from build123d import *

# Parameters (mm, degrees)
F0_W        = 86.36
F0_H        = 24.892
F0_W_2      = 73.66
F0_H_2      = 12.192
F1_DEPTH    = 19.05
F1_FACE_W   = 86.36
F1_FACE_H   = 24.892
F1_FACE_W_2 = 73.66
F1_FACE_H_2 = 12.192
F2_DEPTH    = 12.7
F3_W        = 2.54
F3_H        = 12.192
F3_W_2      = 5.08
F4_DEPTH    = 6.35
F3_W_3      = 86.36
F3_H_2      = 24.892
F5_DEPTH    = 12.7
F7_W        = 73.66
F7_H        = 12.192
F8_DEPTH    = 2.54
F6_W        = 73.66
F6_H        = 3.81
F9_DEPTH    = 18.542


with BuildPart() as f1:
    # F0 (on Top) → F1 (new body)
    with BuildSketch(Plane.XY):
        Rectangle(F0_W, F0_H)
        Rectangle(F0_W_2, F0_H_2, mode=Mode.SUBTRACT)
    extrude(amount=F1_DEPTH)

    # F1_face (on face) → F2 (join)
    with BuildSketch(Plane(origin=(0, 0, 0), x_dir=(1, 0, 0), z_dir=(0, 0, -1))):
        Rectangle(F1_FACE_W, F1_FACE_H)
        Rectangle(F1_FACE_W_2, F1_FACE_H_2, mode=Mode.SUBTRACT)
    extrude(amount=F2_DEPTH)

    # F3 (on face) → F4 (join)
    with BuildSketch(Plane(origin=(0, 0, -12.7), x_dir=(1, 0, 0), z_dir=(0, 0, -1))):
        with Locations((-31.75, 0)):
            Rectangle(F3_W, F3_H)
        Rectangle(F3_W_2, F3_H)
        with Locations((31.75, 0)):
            Rectangle(F3_W, F3_H)
    extrude(amount=-F4_DEPTH)

    # F3 (on face) → F5 (join)
    with BuildSketch(Plane(origin=(0, 0, -12.7), x_dir=(1, 0, 0), z_dir=(0, 0, -1))):
        Rectangle(F3_W_3, F3_H_2)
        Polygon((-2.54, 6.096), (2.54, 6.096), (30.48, 6.096), (33.02, 6.096), (36.83, 6.096), (36.83, -6.096), (33.02, -6.096), (30.48, -6.096), (2.54, -6.096), (-2.54, -6.096), (-30.48, -6.096), (-33.02, -6.096), (-36.83, -6.096), (-36.83, 6.096), (-33.02, 6.096), (-30.48, 6.096), align=None, mode=Mode.SUBTRACT)
    extrude(amount=F5_DEPTH)

    # F7 (on face) → F8 (join)
    with BuildSketch(Plane(origin=(0, 0, -25.4), x_dir=(1, 0, 0), z_dir=(0, 0, -1))):
        Rectangle(F7_W, F7_H)
    extrude(amount=-F8_DEPTH)

    # F6 (on face) → F9 (cut)
    with BuildSketch(Plane.XZ.offset(12.446)):
        with Locations((0, -22.225)):
            Rectangle(F6_W, F6_H)
    extrude(amount=-F9_DEPTH, mode=Mode.SUBTRACT)


solid = f1.part
Here's how the part is built. I have some questions about the finished solid (model axes, mm). A direction names the side the tool comes from. Coordinates: 2 decimals unless noted, no trailing zeros. Order: outer loops, then holes, each group sorted by start corner. A loop starts at its lowest first (then second) coordinate and runs counter-clockwise, first axis right, second up. Notation, with made-up numbers: M 30,-25 L 67,-25 A15 cw 67,-8 Z; hole C 1,87 d1. An arc over 180 degrees is marked long. Answer as CSV lines item,"result".
Item 1: For pin 1 (1 mm diameter, centred on x = -29.5, y = -1, fed in from +Z); pin 2 (1.3 mm diameter, centred on x = -31.5, y = -2.5, fed in from +Z), each with a flat end and sliding along its axis, tell me the tip position at first contact or that it passes through.
Results found:
pin 1,"z = -24.13"
pin 2,"z = -6.35"
Item 2: Imagine slicing it at D-D on x = 0.5. Write out the boundary of the cut face in (y, z), plus the area to 3 significant figures.
Results found:
outline,"M -12.45,-25.4 L 12.45,-25.4 L 12.45,19.05 L 6.1,19.05 L 6.1,-6.35 L -6.1,-6.35 L -6.1,19.05 L -12.45,19.05 L -12.45,-20.32 L -6.1,-20.32 L -6.1,-12.7 L 6.1,-12.7 L 6.1,-24.13 L -12.45,-24.13 Z"
area,"633 mm2"
Item 3: Imagine slicing it at B-B on x = 12. Write out the boundary of the cut face in (y, z), plus the area to 3 significant figures.
Results found:
outline,"M -12.45,-25.4 L 12.45,-25.4 L 12.45,19.05 L 6.1,19.05 L 6.1,-24.13 L -12.45,-24.13 Z; M -12.45,-20.32 L -6.1,-20.32 L -6.1,19.05 L -12.45,19.05 Z"
area,"556 mm2"
Item 4: On a 3-axis mill with a long thin cutter (end or side, diameter ignored), from which of +Z, -Z, +X, -X, +Y, -Y can I reach the whole of each face in a straight line? I mean faces 1 (the face through (33.02, 0, -10)), 2 (the face through (-32, 0, -12.7)), 3 (the face through (-1, 8, 19.05)). Say none if no direction works.
Results found:
face 1,"+Z"
face 2,"none"
face 3,"+Z, +X, -X, +Y, -Y"
Item 5: If I drill on line 1 (X direction, y = -3, z = -11); line 2 (Z direction, x = 1.5, y = -5); line 3 (Y direction, x = -4, z = -5.5), over which ranges is the centre line in solid material (lowest first)?
Results found:
line 1,"-43.18 to -36.83, -33.02 to -30.48, -2.54 to 2.54, 30.48 to 33.02, 36.83 to 43.18"
line 2,"-25.4 to -24.13, -12.7 to -6.35"
line 3,"-12.45 to -6.1, 6.1 to 12.45"
Item 6: We'd pull the mould along Z, two halves only. Please class faces 4 (the face through (-30.48, 0, -10)), 5 (the face through (0, 0, -6.35)), 6 (the face through (0, 0, -12.7)), 7 (the face through (-1, -3, -24.13)): +Z half, -Z half, draft (parallel to the pull), parting line (faces both ways), or undercut.
Results found:
face 4,"draft"
face 5,"+Z half"
face 6,"undercut"
face 7,"undercut"
Item 7: Imagine slicing it at A-A on y = -5. Write out the boundary of the cut face in (x, z), plus the area to 3 significant figures.
Results found:
outline,"M -43.18,-25.4 L 43.18,-25.4 L 43.18,19.05 L 36.83,19.05 L 36.83,-24.13 L -36.83,-24.13 L -36.83,19.05 L -43.18,19.05 Z; M -33.02,-12.7 L -30.48,-12.7 L -30.48,-6.35 L -33.02,-6.35 Z; M -2.54,-12.7 L 2.54,-12.7 L 2.54,-6.35 L -2.54,-6.35 Z; M 30.48,-12.7 L 33.02,-12.7 L 33.02,-6.35 L 30.48,-6.35 Z"
area,"723 mm2"
Item 8: Imagine slicing it at C-C on z = 5.5. Write out the boundary of the cut face in (x, y), plus the area to 3 significant figures.
Results found:
outline,"M -43.18,-12.45 L 43.18,-12.45 L 43.18,12.45 L -43.18,12.45 Z; hole M -36.83,-6.1 L 36.83,-6.1 L 36.83,6.1 L -36.83,6.1 Z"
area,"1,250 mm2"
